For this review, use the dimensioned drawing (mm, ordinates from the lowest corner) and the shaded views. A direction names the side the tool comes from. Round coordinates to 2 decimals unless told otherwise and drop trailing zeros. Loops run counter-clockwise (first coordinate to the right, second up) from the corner with the lowest first, then second, coordinate; pieces in that order, holes last.
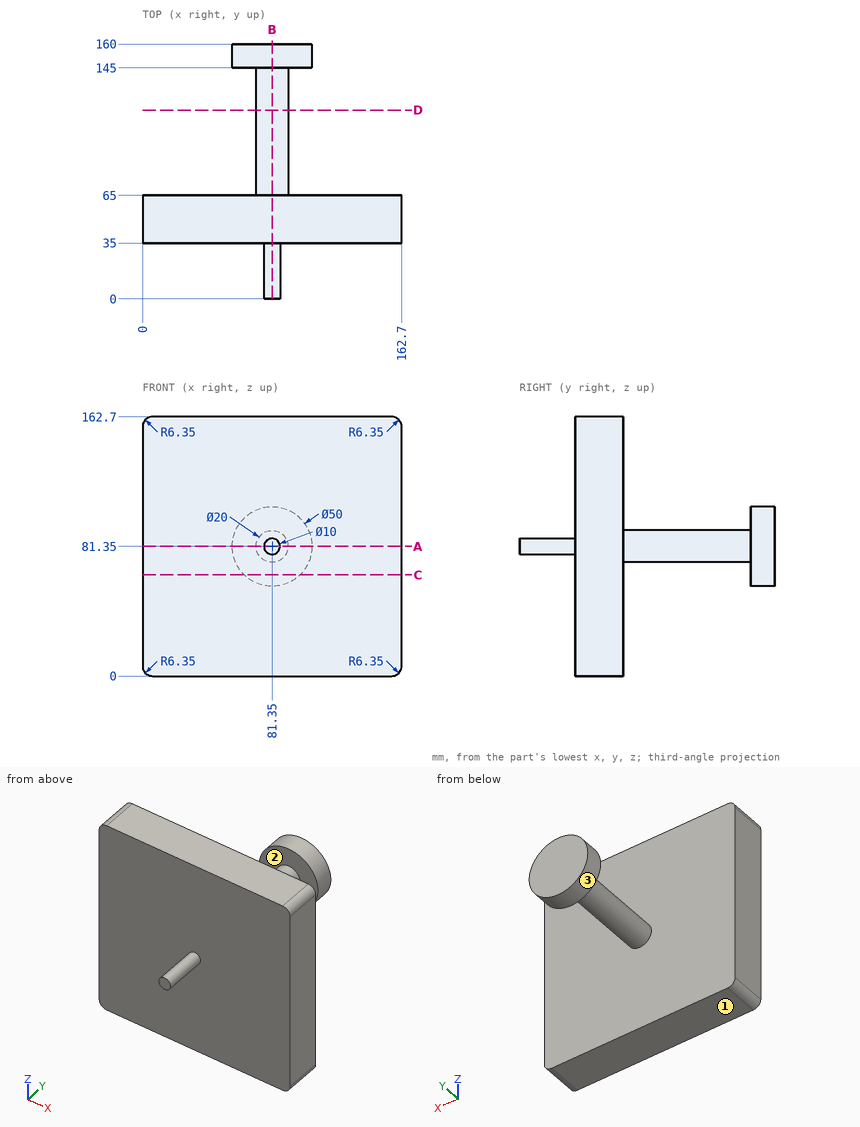
(1) Add section C-C (z = 63.5). Give the boundary of the cut face in (x, y).
(2) Add section A-A (z = 81.35). Give the boundary of the cut face in (x, y).
(3) For the marked faces 1, 2 and 3, list the 3-axis set-ups (+Z, -Z, +X, -X, +Y, -Y) from which the entire face can be reached by the end or side of a thin tool; tool diameter is ignored.
(4) Add section B-B (x = 81.35). Give the boundary of the cut face in (y, z).
(5) For L1, parallel to Y at x = 72, z = 65.5; L2, parallel to Y at x = 47, z = 127; L3, parallel to Y at x = 89, z = 77, list the stretches that pass through material, from the lowest coordinate up.
(6) Insertion check: pin 1 Ø4 at (x, z) = (20, 19.5) entering from -Y; pin 2 Ø1.5 at (y, z) = (95.5, 84) entering from +X; pin 3 Ø8 at (y, z) = (106, 71.5) entering from -X; pin 4 Ø12 at (x, y) = (101.5, 101) entering from +Z. Each pin has a flat end and moves straight along its axis. Give the tip position at first contact, or say it passes through.
(7) Add section D-D (y = 118.5). Give the boundary of the cut face in (x, z), plus the area to 3 significant figures.
Outcome:
1. outline: (0, 35) - (162.7, 35) - (162.7, 65) - (0, 65) - close; (63.85, 145) - (98.85, 145) - (98.85, 160) - (63.85, 160) - close
2. outline: (0, 35) - (76.35, 35) - (76.35, 0) - (86.35, 0) - (86.35, 35) - (162.7, 35) - (162.7, 65) - (91.35, 65) - (91.35, 145) - (106.35, 145) - (106.35, 160) - (56.35, 160) - (56.35, 145) - (71.35, 145) - (71.35, 65) - (0, 65) - close
3. face 1: -Z, +X, -X, +Y, -Y
3. face 2: none
3. face 3: +Y
4. outline: (0, 76.35) - (35, 76.35) - (35, 0) - (65, 0) - (65, 71.35) - (145, 71.35) - (145, 56.35) - (160, 56.35) - (160, 106.35) - (145, 106.35) - (145, 91.35) - (65, 91.35) - (65, 162.7) - (35, 162.7) - (35, 86.35) - (0, 86.35) - close
5. L1: y = 35 to 65, 145 to 160
5. L2: y = 35 to 65
5. L3: y = 35 to 160
6. pin 1: stops at y = 35
6. pin 2: stops at x = 91.17
6. pin 3: stops at x = 73.24
6. pin 4: passes through
7. outline: circle Ø20 at (81.35, 81.35)
7. area: 314 mm2
